Work out the finished part from the listing and answer in its coordinate system (mm). Face numbers are marked on the shaded views. A direction names the side the tool comes from. Give positions to 0.01 mm unless a question says otherwise; leave off trailing zeros. Order: outer loops, then holes, each group sorted by start corner. A loop starts at its lowest first (then second) coordinate and runs counter-clockwise, first axis right, second up. Notation, with made-up numbers: (-12, 28) - (14, 28) arc R21 ccw to (14, 52) - close; hole circle Ø2 at (56, -19.75). An arc over 180 degrees is marked (long way). Return JSON: item names as keys, results as strings. Group by question number.
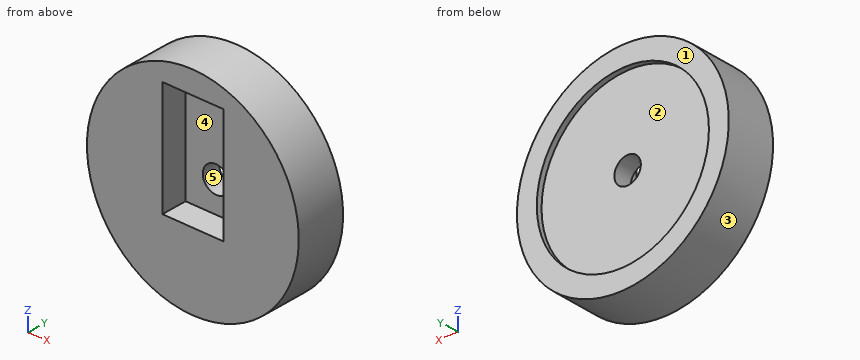
from build123d import *

# Parameters (mm, degrees)
SKETCH1_R               = 40
BOSS_EXTRUDE1_DEPTH     = 18.75
SKETCH1_3_W             = 23
SKETCH1_3_H             = 43
CUT_EXTRUDE1_DEPTH      = 9.8
CUT_EXTRUDE2_DEPTH      = 60.594987205
CUT_EXTRUDE2_DEPTH_BACK = 60.594987205
SKETCH1_4_R             = 5
CUT_EXTRUDE3_START      = 18.75
SKETCH1_5_R             = 32.5
CUT_EXTRUDE3_DEPTH      = 2


with BuildPart() as part:
    # Sketch1 → Boss-Extrude1 (new body)
    with BuildSketch(Plane(origin=(0, 0, 0), x_dir=(1, 0, 0), z_dir=(0, 1, 0))):
        with Locations(Location((0, 0, 0), (0, 0, 270))):
            Circle(SKETCH1_R)
    extrude(amount=BOSS_EXTRUDE1_DEPTH)

    # Sketch1<3> → Cut-Extrude1 (cut)
    with BuildSketch(Plane(origin=(0, 0, 0), x_dir=(1, 0, 0), z_dir=(0, 1, 0))):
        with Locations((0, -10)):
            Rectangle(SKETCH1_3_W, SKETCH1_3_H)
    extrude(amount=CUT_EXTRUDE1_DEPTH, mode=Mode.SUBTRACT)

    # Sketch1<4> → Cut-Extrude2 (cut, two sides: drawn at the far end of the back side and taken through both)
    with BuildSketch(Plane(origin=(0, 0, 0), x_dir=(1, 0, 0), z_dir=(0, 1, 0)).offset(-CUT_EXTRUDE2_DEPTH_BACK)):
        with Locations(Location((0, 0, 0), (0, 0, 270))):
            Circle(SKETCH1_4_R)
    extrude(amount=CUT_EXTRUDE2_DEPTH + CUT_EXTRUDE2_DEPTH_BACK, mode=Mode.SUBTRACT)

    # Sketch1<5> → Cut-Extrude3 (cut)
    with BuildSketch(Plane(origin=(0, 0, 0), x_dir=(1, 0, 0), z_dir=(0, 1, 0)).offset(CUT_EXTRUDE3_START)):
        with Locations(Location((0, 0, 0), (0, 0, 270))):
            Circle(SKETCH1_5_R)
    extrude(amount=-CUT_EXTRUDE3_DEPTH, mode=Mode.SUBTRACT)


solid = part.part
1. The part is cut by section C-C (y = 2). Give the vertices of the cut face in (x, z), and give its area (3 significant figures).
2. Determine the mould class of the marked faces 1, 2 and 3 for opening direction X: released by +X, released by -X, zero draft, split by the parting line, or undercut.
3. Consider probe 1 along Y at (x, z) = (17, -13.5); probe 2 along X at (y, z) = (13, 0). Determine where each line is inside the solid, lowest interval first. Write a range as from..to.
4. A tool of negligible diameter and unlimited length cuts with its end or side. For the marked faces 4 and 5, from which of +Z, -Z, +X, -X, +Y, -Y can it reach the whole face along a straight path? Write none if from no direction.
5. The part is cut by section B-B (x = 0). Give the vertices of the cut face in (y, z).
6. Each of these flat-tipped pins is pushed along its axis until it touches: pin 1 (1 mm diameter, centred on x = 20.5, y = 8.5, fed in from +Z); pin 2 (5 mm diameter, centred on x = -30.5, y = 7.5, fed in from -Z); pin 3 (1 mm diameter, centred on y = 14.5, z = -14, fed in from -X). Where does it stop, or does it pass through?
7. The part is cut by section D-D (z = -28.5). Give the vertices of the cut face in (x, y), and give its area (3 significant figures).
8. The part is cut by section A-A (z = 0). Give the vertices of the cut face in (x, y).
Answers:
{
 "1": {"outline": "circle Ø80 at (0, 0); hole (-11.5, -11.5) - (11.5, -11.5) - (11.5, 31.5) - (-11.5, 31.5) - close", "area": "4,040 mm^2"},
 "2": {"face 1": "zero draft", "face 2": "undercut", "face 3": "split by the parting line"},
 "3": {"probe 1": "y = 0..16.75", "probe 2": "x = -40..-5, 5..40"},
 "4": {"face 4": "-Y", "face 5": "+Y, -Y"},
 "5": {"outline": "(0, -40) - (18.75, -40) - (18.75, -32.5) - (16.75, -32.5) - (16.75, -5) - (9.8, -5) - (9.8, -11.5) - (0, -11.5) - close; (0, 31.5) - (9.8, 31.5) - (9.8, 5) - (16.75, 5) - (16.75, 32.5) - (18.75, 32.5) - (18.75, 40) - (0, 40) - close"},
 "6": {"pin 1": "stops at z = 34.64", "pin 2": "stops at z = -28.57", "pin 3": "stops at x = -37.65"},
 "7": {"outline": "(-28.07, 0) - (28.07, 0) - (28.07, 18.75) - (15.62, 18.75) - (15.62, 16.75) - (-15.62, 16.75) - (-15.62, 18.75) - (-28.07, 18.75) - close", "area": "990 mm^2"},
 "8": {"outline": "(-40, 0) - (-11.5, 0) - (-11.5, 9.8) - (-5, 9.8) - (-5, 16.75) - (-32.5, 16.75) - (-32.5, 18.75) - (-40, 18.75) - close; (5, 9.8) - (11.5, 9.8) - (11.5, 0) - (40, 0) - (40, 18.75) - (32.5, 18.75) - (32.5, 16.75) - (5, 16.75) - close"}
}
